The model under review builds one solid part; all positions refer to its coordinate system, in mm. A direction names the side the tool comes from. Coordinates: 2 decimals unless noted, no trailing zeros. Write each loop counter-clockwise with the first axis right and the second up, starting at its lowest first coordinate (ties: lowest second). Pieces come first, ordered by that corner, then holes.
1) Add section A-A, the plane y = 0. State the section outline as (x, z) points.
2) Mouldability with a two-part tool opening along Y and no side actions: class faces 1 (the cylindrical face through (-6.324, -41.853, 4.93)), 2 (the cylindrical face through (-1.301, 19.143, 5.07)), 3 (the cylindrical face through (-69.27, -0.11, 22.44)) as released by +Y, released by -Y, zero draft, split by the parting line, or undercut.
3) Add section C-C, the plane z = 30. State the section outline as (x, y) points, then the cut area to 3 significant figures.
4) For P1, Ø1, axis at y = -14.5, z = 11, coming from the -X side; P2, Ø3, axis at y = 18.5, z = 3.5, coming from the -X side; P3, Ø3, axis at x = -57, z = 10, coming from the -Y side; P4, Ø5, axis at x = -42, z = 19, coming from the +Y side, all flat-tipped, find the tip position at first contact; note any pin that passes through.
5) Add section D-D, the plane x = -57. State the section outline as (y, z) points.
6) For line 1 (Y direction, x = 0, z = 4); line 2 (Z direction, x = 32, y = -21); line 3 (Z direction, x = -67.5, y = -2.5), list the stretches that pass through material, from the lowest coordinate up.
7) Machinability: for faces 4 (the cylindrical face through (-5.74, 42.06, 4.93)), 5 (the flat face through (-18, -16, 5)), 6 (the flat face through (-18, 17, 5)), which of the approach directions +Z, -Z, +X, -X, +Y, -Y give a long, thin tool a straight path to every point of the face, cutting with its end or side? Answer none if there is none.
8) Add section B-B, the plane x = 0. State the section outline as (y, z) points.
from build123d import *

# Parameters (mm, degrees)
F1_DEPTH = 10
F3_DEPTH = 8
F4_R     = 125
F6_R     = 6
F7_DEPTH = 25
F8_R     = 10
F9_DEPTH = 25


with BuildPart() as f1:
    # F0 (on Top) → F1 (new body)
    with BuildSketch(Plane.XY):
        with BuildLine():
            ThreePointArc((13.956018, -36.367918), (30.362055, -23.224109), (50.720724, -17.985565))
            ThreePointArc((50.720724, -17.985565), (68, 0), (50.720724, 17.985565))
            ThreePointArc((50.720724, 17.985565), (30.362055, 23.224109), (13.956018, 36.367918))
            ThreePointArc((13.956018, 36.367918), (-6.032896, 41.958896), (-18, 25))
            Line((-18, 25), (-18, -25))
            ThreePointArc((-18, -25), (-6.032896, -41.958896), (13.956018, -36.367918))
        make_face()
    extrude(amount=F1_DEPTH)


with BuildPart() as f3:
    # F2 (on Front) → F3 (new body, symmetric)
    with BuildSketch(Plane.XZ):
        with BuildLine():
            Line((-59.279276, 0), (50.720724, 0))
            Line((50.720724, 0), (50.720724, 10))
            Line((50.720724, 10), (-40.840187, 10))
            ThreePointArc((-40.840187, 10), (-69.767365, 41.33908), (-59.279276, 0))
        make_face()
    extrude(amount=F3_DEPTH, both=True)

    # F4
    f4_edges = [f3.edges().sort_by_distance(p)[0] for p in [
        (-40.840187, 0, 10),
    ]]
    fillet(f4_edges, radius=F4_R)

    # F5: union F1
    add(f1.part)

    # F6 (on face) → F7 (cut)
    with BuildSketch(Plane.XY.offset(10)):
        with Locations((0, 25)):
            Circle(F6_R)
        with Locations((0, -25)):
            Circle(F6_R)
        with Locations((50, 0)):
            Circle(F6_R)
    extrude(amount=-F7_DEPTH, mode=Mode.SUBTRACT)

    # F8 (on face) → F9 (cut)
    with BuildSketch(Plane.XZ.offset(8)):
        with Locations((-59.279276, 22)):
            Circle(F8_R)
    extrude(amount=-F9_DEPTH, mode=Mode.SUBTRACT)


solid = f3.part
Geometry results:
1. outline: (-59.28, 0) - (44, 0) - (44, 10) - (34.74, 10) arc R125 cw to (-45.21, 38.91) arc R22 ccw (long way) to start; (56, 0) - (68, 0) - (68, 10) - (56, 10) - close; hole circle Ø20 at (-59.28, 22)
2. face 1: released by -Y
2. face 2: undercut
2. face 3: zero draft
3. outline: (-79.77, -8) - (-65.28, -8) - (-65.28, 8) - (-79.77, 8) - close; (-53.28, -8) - (-33.08, -8) - (-33.08, 8) - (-53.28, 8) - close
3. area: 555 mm2
4. P1: passes through
4. P2: stops at x = -18
4. P3: stops at y = -8
4. P4: stops at y = 8
5. outline: (-8, 0) - (8, 0) - (8, 12.26) - (-8, 12.26) - close; (-8, 31.74) - (8, 31.74) - (8, 43.88) - (-8, 43.88) - close
6. line 1: y = -43 to -31, -19 to 19, 31 to 43
6. line 2: z = 0 to 10
6. line 3: z = 1.59 to 16.31, 27.69 to 42.41
7. face 4: +Z, -Z, +Y
7. face 5: +Z, -Z, -X, -Y
7. face 6: +Z, -Z, -X, +Y
8. outline: (-43, 0) - (-31, 0) - (-31, 10) - (-43, 10) - close; (-19, 0) - (19, 0) - (19, 10) - (8, 10) - (8, 14.93) - (-8, 14.93) - (-8, 10) - (-19, 10) - close; (31, 0) - (43, 0) - (43, 10) - (31, 10) - close
